Model file for the job. Use its own axes, mm. Coordinates: 2 decimals unless noted, no trailing zeros. Loops run counter-clockwise (first coordinate to the right, second up) from the corner with the lowest first, then second, coordinate; pieces in that order, holes last. Notation, with made-up numbers: (78, -4.5) - (105, -4.5) arc R29 ccw to (105, 25.5) - close; hole circle Ø7 at (-32, 20). An arc over 180 degrees is marked (long way). Write each question's results on one line, items separated by ' | '. Start each with the question number.
```python
from build123d import *

# Parameters (mm, degrees)
BASE_FLANGE1_DEPTH                            = 2.286
CSK_FOR_8_FLAT_HEAD_MACHINE_SCREW1_AT_2_COUNT = 2
CSK_FOR_8_FLAT_HEAD_MACHINE_SCREW1_AT_2_PITCH = 20.32


# Sheet-metal steps are written as plain solids
with BuildPart() as part:
    # Sketch1 → Base-Flange1 (new body)
    with BuildSketch(Plane.XY):
        with BuildLine():
            Line((10.16, -5.715), (-10.16, -5.715))
            ThreePointArc((-10.16, -5.715), (-15.875, 0), (-10.16, 5.715))
            Line((-10.16, 5.715), (10.16, 5.715))
            ThreePointArc((10.16, 5.715), (15.875, 0), (10.16, -5.715))
        make_face()
    extrude(amount=-BASE_FLANGE1_DEPTH)

    # Sketch4 → CSK for #8 Flat Head Machine Screw1 (revolve, cut)
    with BuildSketch(Plane(origin=(-10.16, 0, 0), x_dir=(0, -1, 0), z_dir=(1, 0, 0))):
        Polygon((0, 0), (0, 2.286), (2.2479, 2.286), (2.2479, 2.77249335), (4.6579917, 0), align=None)
    csk_for_8_flat_head_machine_screw1 = revolve(axis=Axis((-10.16, 0, 6.35), (0, 0, -1)), mode=Mode.SUBTRACT)

    # CSK for #8 Flat Head Machine Screw1 at 2: CSK for #8 Flat Head Machine Screw1 ×2
    with Locations(*[(i * CSK_FOR_8_FLAT_HEAD_MACHINE_SCREW1_AT_2_PITCH, 0, 0) for i in range(1, CSK_FOR_8_FLAT_HEAD_MACHINE_SCREW1_AT_2_COUNT)]):
        add(csk_for_8_flat_head_machine_screw1, mode=Mode.SUBTRACT)


solid = part.part
```
Q1. Mould opens along X. For faces 1 (the cylindrical face through (15.874, 0.126, -1.127)), 2 (the conical face through (9.3, -2.7, -2.1)), 3 (the flat face through (0, -5.715, -1)) say: +X half, -X half, draft (parallel to the pull), parting line (faces both ways), or undercut.
Q2. Cut at A-A (y = 0). List the corners of the cut face in (x, z) (3 decimals).
Q3. Drill centre lines: L1, parallel to X at y = 2.5, z = -1; L2, parallel to X at y = -0.75, z = -0.6; L3, parallel to Y at x = 8, z = -1.5 (3 decimals). Where is each one in solid material? Low to high. Write a range as from..to.
Q4. Pin check, flat tip, straight feed: pin 1 (1 mm diameter, centred on y = 4, z = -1.5, fed in from -X). Stop position of the tip, or through.
Q5. Cut at B-B (z = -1.2). List the corners of the cut face in (x, y) (3 decimals), and give its area (3 significant figures).
Check result:
1) face 1: +X half | face 2: undercut | face 3: draft
2) outline: (-15.875, -2.286) - (-12.831, -2.286) - (-14.818, 0) - (-15.875, 0) - close; (-7.489, -2.286) - (7.489, -2.286) - (5.502, 0) - (-5.502, 0) - close; (12.831, -2.286) - (15.875, -2.286) - (15.875, 0) - (14.818, 0) - close
3) L1: -15.3..-13.01, -7.31..7.31, 13.01..15.3 | L2: -15.83..-14.23, -6.09..6.09, 14.23..15.83 | L3: -5.715..-2.566, 2.566..5.715
4) pin 1: x = -14.68
5) outline: (-10.16, -5.715) - (10.16, -5.715) arc R5.715 ccw to (10.16, 5.715) - (-10.16, 5.715) arc R5.715 ccw to start; hole circle Ø7.23 at (-10.16, 0); hole circle Ø7.23 at (10.16, 0) | area: 253 mm²
